Work out the finished part from the listing and answer in its coordinate system (mm). A direction names the side the tool comes from. Coordinates: 2 decimals unless noted, no trailing zeros. Order: outer loops, then holes, each group sorted by start corner. A loop starts at its lowest first (then second) coordinate and runs counter-clockwise, first axis right, second up.
1. Determine the mould class of faces 1 (the flat face through (42, 84, -3)), 2 (the flat face through (-15.111, 37.315, -241.621)), 3 (the flat face through (18.36, 55.48, 237.05)), 4 (the cylindrical face through (-43.014, 29.993, -0.66)) for opening direction Z: +Z half, -Z half, draft (parallel to the pull), parting line (faces both ways), or undercut.
2. The part is cut by section A-A, the plane z = 0. Give the vertices of the cut face in (x, y), then the cut area to 3 significant figures.
3. A tool of negligible diameter and unlimited length cuts with its end or side. For faces 5 (the cylindrical face through (42.986, 29.993, -0.66)), 6 (the flat face through (-44, 86, -3)), 7 (the flat face through (-42, 86, -3)), 8 (the flat face through (44, 84, -3)), from which of +Z, -Z, +X, -X, +Y, -Y can it reach the whole face along a straight path? Write none if from no direction.
4. The part is cut by section B-B, the plane x = -33.5. Give the vertices of the cut face in (y, z), then the cut area to 3 significant figures.
5. Find the intervals of material crossed by probe 1 along X at (y, z) = (148.5, -55); probe 2 along X at (y, z) = (117.5, 181.5); probe 3 along Z at (x, y) = (33, 171), in increasing order.
6. The part is cut by section C-C, the plane x = -3. Give the vertices of the cut face in (y, z).
7. Flat-ended cylindrical pins translate along their axes: pin 1 Ø4 at (x, z) = (-16, 53.5) entering from +Y; pin 2 Ø1.5 at (x, y) = (10, 101.5) entering from -Z; pin 3 Ø12 at (x, z) = (-37.5, 104) entering from +Y. Find the tip coordinate at first contact, or state that the pin passes through.
```python
from build123d import *

# Parameters (mm, degrees)
CUT_EXTRUDE1_DEPTH      = 355.271082801
CUT_EXTRUDE1_DEPTH_BACK = 355.271082801
SHELL1_T                = -2


with BuildPart() as part:
    # Sketch1 → Revolve1 (revolve)
    with BuildSketch(Plane.XY, mode=Mode.PRIVATE) as revolve1_sk:
        with BuildLine():
            Line((-44, 0), (44, 0))
            Line((44, 0), (44, 170))
            ThreePointArc((44, 170), (44.406955742, 173.841366627), (45.609756098, 177.512195122))
            ThreePointArc((45.609756098, 177.512195122), (0, 248), (-45.609756098, 177.512195122))
            ThreePointArc((-45.609756098, 177.512195122), (-44.406955742, 173.841366627), (-44, 170))
            Line((-44, 170), (-44, 0))
        make_face()
    revolve(revolve1_sk.sketch.rotate(Axis((-44, 0, 0), (1, 0, 0)), 180), axis=Axis((-44, 0, 0), (1, 0, 0)))

    # Sketch2 → Cut-Extrude1 (cut, two sides: drawn at the far end of the back side and taken through both)
    with BuildSketch(Plane(origin=(0, 0, 0), x_dir=(0, 0, -1), z_dir=(1, 0, 0)).offset(-CUT_EXTRUDE1_DEPTH_BACK)):
        with BuildLine():
            Line((-30, 0), (-289.335468676, 69.4887294))
            Line((-289.335468676, 69.4887294), (-289.335468676, -330.5112706))
            Line((-289.335468676, -330.5112706), (310.664531324, -330.5112706))
            Line((310.664531324, -330.5112706), (310.664531324, 49.4887294))
            Line((310.664531324, 49.4887294), (30, 0))
            ThreePointArc((30, 0), (0, 30), (-30, 0))
        make_face()
    extrude(amount=CUT_EXTRUDE1_DEPTH + CUT_EXTRUDE1_DEPTH_BACK, mode=Mode.SUBTRACT)

    # Shell1
    shell1_openings = [part.faces().sort_by_distance(p)[0] for p in [
        (1.12e-07, 18.550551002, -135.20540264),
        (-1.736e-06, 27.714135748, 133.430562698),
        (0, 30, 0),
    ]]
    offset(amount=SHELL1_T, openings=shell1_openings, kind=Kind.INTERSECTION)


solid = part.part
```
Geometry says:
1. face 1: undercut
1. face 2: -Z half
1. face 3: +Z half
1. face 4: undercut
2. outline: (-45.61, 177.51) arc R18.33 cw to (-44, 170) - (-44, 30) - (-42, 30) - (-42, 170) arc R20.33 ccw to (-43.79, 178.33) arc R48 cw (long way) to (43.79, 178.33) arc R20.33 ccw to (42, 170) - (42, 30) - (44, 30) - (44, 170) arc R18.33 cw to (45.61, 177.51) arc R50 ccw (long way) to start
2. area: 983 mm2
3. face 5: +X, -X, -Y
3. face 6: -X, -Y
3. face 7: -Y
3. face 8: +X, -Y
4. outline: (35.21, -229.69) - (35.69, -232.39) arc R235.12 ccw to (53.32, 228.99) - (52.61, 226.34) arc R232.38 cw to start
4. area: 1,770 mm2
5. probe 1: x = -44 to -42, 42 to 44
5. probe 2: x = -46.56 to -44.41, 44.41 to 46.56
5. probe 3: z = -162.02 to -158.05, 158.05 to 162.02
6. outline: (37.56, -243.02) - (37.91, -244.99) arc R247.91 ccw to (56.63, 241.35) - (56.11, 239.42) arc R245.91 cw to start
7. pin 1: stops at y = 240.26
7. pin 2: stops at z = -225.55
7. pin 3: stops at y = 213.49
